Autodesk Inventor part; units mm, degrees
ref_plane "YZ Plane" through (0, 0, 0) normal (1, 0, 0) x (0, 1, 0)
ref_plane "XZ Plane" through (0, 0, 0) normal (0, 1, 0) x (-1, 0, 0)
ref_plane "XY Plane" through (0, 0, 0) normal (0, 0, 1) x (1, 0, 0)
sketch "Sketch1" plane through (0, 0, 0) normal (0, 1, 0) x (-1, 0, 0)
  line L0 (0, -5.4) -> (1.5, -5.4)
  line L1 (1.5, -5.4) -> (1.5, -8.1)
  line L2 (1.5, -8.1) -> (3.2, -8.1)
  line L3 (0, 0) -> (1.5, 0)
  line L4 (1.5, 0) -> (1.5, 2.7)
  line L5 (1.5, 2.7) -> (3.2, 2.7)
  line L6 (5, 0) -> (5, -5.4)
  line L7 (5, -5.4) -> (3.2, -8.1)
  line L8 (5, 0) -> (3.2, 2.7)
  line L9 (0, -20) -> (1.5, -20)
  line L10 (1.5, -20) -> (1.5, -17.3)
  line L11 (1.5, -17.3) -> (3.2, -17.3)
  line L12 (0, -25.4) -> (1.5, -25.4)
  line L13 (1.5, -25.4) -> (1.5, -28.1)
  line L14 (1.5, -28.1) -> (3.2, -28.1)
  line L15 (5, -20) -> (5, -25.4)
  line L16 (5, -25.4) -> (3.2, -28.1)
  line L17 (5, -20) -> (3.2, -17.3)
  line L18 (0, -5.4) -> (0, -20)
  line L19 (0, 0) -> (0, 7.3)
  line L20 (0, 7.3) -> (-5, 7.3)
  line L21 (0, -25.4) -> (0, -32.7)
  line L22 (0, -32.7) -> (-5, -32.7)
  line L23 (-5, -32.7) -> (-5, 7.3)
  dimension "d0" = 5.4
  dimension "d1" = 1.5
  dimension "d2" = 2.7
  dimension "d3" = 1.7
  dimension "d4" = 2.7
  dimension "d5" = 1.7
  dimension "d9" = 2.7
  dimension "d10" = 2.7
  dimension "d11" = 5.4
  dimension "d12" = 7.3
  dimension "d13" = 5
  dimension "d14" = 7.3
  dimension "d15" = 5
  dimension "d16" = 20
extrude "Extrusion1" add sketch "Sketch1" along normal blind 40
sketch "Sketch2" plane through (5, 0, 7.3) normal (1, 0, 0) x (0, 0, -1)
  line L0 (11.6599, 5) -> (8.3401, 5)
  line L1 (8.3401, 5) -> (6.6802, 7.875)
  line L2 (6.6802, 7.875) -> (8.3401, 10.75)
  line L3 (8.3401, 10.75) -> (11.6599, 10.75)
  line L4 (11.6599, 10.75) -> (13.3198, 7.875)
  line L5 (13.3198, 7.875) -> (11.6599, 5)
  line L6 (40, 0) -> (0, 0)
  line L7 (0, 0) -> (0, 40)
  line L8 (31.6599, 5) -> (28.3401, 5)
  line L9 (28.3401, 5) -> (26.6802, 7.875)
  line L10 (26.6802, 7.875) -> (28.3401, 10.75)
  line L11 (28.3401, 10.75) -> (31.6599, 10.75)
  line L12 (31.6599, 10.75) -> (33.3198, 7.875)
  line L13 (33.3198, 7.875) -> (31.6599, 5)
  line L14 (40, 0) -> (40, 40)
  line L15 (11.6599, 29.25) -> (8.3401, 29.25)
  line L16 (8.3401, 29.25) -> (6.6802, 32.125)
  line L17 (6.6802, 32.125) -> (8.3401, 35)
  line L18 (8.3401, 35) -> (11.6599, 35)
  line L19 (11.6599, 35) -> (13.3198, 32.125)
  line L20 (13.3198, 32.125) -> (11.6599, 29.25)
  line L21 (31.6599, 29.25) -> (28.3401, 29.25)
  line L22 (28.3401, 29.25) -> (26.6802, 32.125)
  line L23 (26.6802, 32.125) -> (28.3401, 35)
  line L24 (28.3401, 35) -> (31.6599, 35)
  line L25 (31.6599, 35) -> (33.3198, 32.125)
  line L26 (33.3198, 32.125) -> (31.6599, 29.25)
  line L27 (0, 40) -> (40, 40)
  point P0 (7.3, 0)
  point P1 (10, 7.875)
  point P2 (30, 7.875)
  point P3 (10, 32.125)
  point P4 (30, 32.125)
  dimension "d17" = 5.75
  dimension "d18" = 5
  dimension "d19" = 10
  dimension "d20" = 5.75
  dimension "d21" = 5
  dimension "d22" = 10
  dimension "d23" = 5.75
  dimension "d24" = 5.75
  dimension "d25" = 5
  dimension "d26" = 5
  dimension "d27" = 10
  dimension "d28" = 10
extrude "Extrusion2" cut sketch "Sketch2" against normal blind 2.5 contours L0 L1 L2 L3 L4 L5 | L8 L9 L10 L11 L12 L13 | L15 L16 L17 L18 L19 L20 | L21 L22 L23 L24 L25 L26
sketch "Sketch3" plane through (2.5, 0, 7.3) normal (1, 0, 0) x (0, 0, -1)
  circle A0 centre (30, 7.75) radius 1.375
  circle A1 centre (10, 7.75) radius 1.375
  circle A2 centre (10, 32.25) radius 1.375
  circle A3 centre (30, 32.25) radius 1.375
  point P0 (7.3, 0)
  dimension "d31" = 2.75
  dimension "d32" = 2.75
  dimension "d33" = 2.75
extrude "Extrusion3" cut sketch "Sketch3" against normal blind 20
sketch "Sketch4" plane through (0, 40, 0) normal (0, 1, 0) x (1, 0, 0)
  line L0 (5, -7.3) -> (5, 32.7)
  line L1 (5, -7.3) -> (-55, -7.3)
  line L2 (-55, -7.3) -> (-55, 32.7)
  line L3 (-55, 32.7) -> (5, 32.7)
  line L4 (5, 32.7) -> (5, -7.3)
  point P0 (0, 0)
  dimension "d36" = 60
extrude "Extrusion4" add sketch "Sketch4" along normal blind 5
sketch "Sketch5" plane through (0, 40, 0) normal (0, -1, 0) x (1, 0, 0)
  line L0 (-55, -32.7) -> (-55, 7.3)
  line L1 (-20.2, 0) -> (-55, 0)
  line L2 (-55, 0) -> (-55, -5.4)
  line L3 (-55, -5.4) -> (-20.2, -5.4)
  line L4 (-20.2, -5.4) -> (-20.2, 0)
  line L5 (0, -5.4) -> (0, -20)
  line L6 (-20.2, -20) -> (-55, -20)
  line L7 (-55, -20) -> (-55, -25.4)
  line L8 (-55, -25.4) -> (-20.2, -25.4)
  line L9 (-20.2, -25.4) -> (-20.2, -20)
  point P0 (0, 0)
  dimension "d39" = 5.4
  dimension "d40" = 20.2
  dimension "d41" = 5.4
extrude "Extrusion5" add sketch "Sketch5" along normal blind 1.5
sketch "Sketch6" plane through (-55, 40, 7.3) normal (-1, 0, 0) x (0, 0, 1)
  point P0 (-7.3, -40)
sketch "Sketch7" plane through (-55, 40, 7.3) normal (-1, 0, 0) x (0, 0, 1)
  point P0 (-7.3, -40)
sketch "Sketch8" plane through (0, 38.5, 0) normal (0, -1, 0) x (1, 0, 0)
  line L0 (-55, -32.7) -> (-55, 7.3)
  line L1 (-20.2, 2.7) -> (-55, 2.7)
  line L2 (-55, 2.7) -> (-55, -8.1)
  line L3 (-55, -8.1) -> (-20.2, -8.1)
  line L4 (-20.2, -8.1) -> (-20.2, 2.7)
  line L5 (-20.2, -17.3) -> (-55, -17.3)
  line L6 (-55, -17.3) -> (-55, -28.1)
  line L7 (-55, -28.1) -> (-20.2, -28.1)
  line L8 (-20.2, -28.1) -> (-20.2, -17.3)
  line L9 (-20.2, -20) -> (-55, -20)
  point P0 (0, 0)
  dimension "d44" = 10.8
  dimension "d45" = 10.8
  dimension "d46" = 2.7
extrude "Extrusion6" add sketch "Sketch8" along normal blind 1.7 contours L0 L1 L4 L3 | L0 L9 L8 L7
sketch "Sketch9" plane through (-55, 40, 7.3) normal (-1, 0, 0) x (0, 0, 1)
  line L0 (-7.3, -4.809) -> (-12.7, -4.809)
  line L1 (-12.7, -40) -> (-12.7, 0)
  line L2 (-4.6, -3.2) -> (-15.4, -3.2)
  line L3 (-12.7, -4.809) -> (-15.4, -3.2)
  line L4 (-15.4, -3.2) -> (-4.6, -3.2)
  line L5 (-4.6, -3.2) -> (-7.3, -4.809)
  point P0 (-7.3, -40)
  dimension "d49" = 5.4
extrude "Extrusion7" add sketch "Sketch9" against normal blind 34.8
sketch "Sketch10" plane through (-55, 40, -20) normal (0, 0, 1) x (1, 0, 0)
  line L0 (34.8, -3.2) -> (0, -3.2)
  line L1 (0, 0) -> (0, -3.2)
  line L2 (34.8, -3.2) -> (0, -3.2)
  line L3 (0, -3.2) -> (0, -1.5)
  line L4 (0, -1.5) -> (34.8, -1.5)
  line L5 (34.8, -1.5) -> (34.8, -3.2)
  point P0 (55, -40)
  dimension "d52" = 1.7
extrude "Extrusion8" add sketch "Sketch10" along normal blind 2.7
sketch "Sketch11" plane through (-55, 40, 7.3) normal (-1, 0, 0) x (0, 0, 1)
  line L0 (-24.6, -3.2) -> (-24.6, -1.5)
  line L1 (-35.4, -3.2) -> (-24.6, -3.2)
  line L2 (-24.6, -3.2) -> (-35.4, -3.2)
  line L3 (-27.3, -5) -> (-32.7, -5)
  line L4 (-32.7, -5) -> (-35.4, -3.2)
  line L5 (-24.6, -3.2) -> (-27.3, -5)
  line L6 (-27.3, 0) -> (-32.7, 0)
  point P0 (-7.3, -40)
  dimension "d55" = 5.4
  dimension "d56" = 5
extrude "Extrusion9" add sketch "Sketch11" against normal blind 34.8
sketch "Sketch12" plane through (0, 45, 0) normal (0, 1, 0) x (1, 0, 0)
  line L0 (-44.25, 4.3599) -> (-44.25, 1.0401)
  line L1 (-44.25, 1.0401) -> (-47.125, -0.6198)
  line L2 (-47.125, -0.6198) -> (-50, 1.0401)
  line L3 (-50, 1.0401) -> (-50, 4.3599)
  line L4 (-50, 4.3599) -> (-47.125, 6.0198)
  line L5 (-47.125, 6.0198) -> (-44.25, 4.3599)
  line L6 (-44.25, 24.3599) -> (-44.25, 21.0401)
  line L7 (-44.25, 21.0401) -> (-47.125, 19.3802)
  line L8 (-47.125, 19.3802) -> (-50, 21.0401)
  line L9 (-50, 21.0401) -> (-50, 24.3599)
  line L10 (-50, 24.3599) -> (-47.125, 26.0198)
  line L11 (-47.125, 26.0198) -> (-44.25, 24.3599)
  line L12 (-55, 25.4) -> (-20.2, 25.4)
  line L13 (-29.25, 4.3599) -> (-29.25, 1.0401)
  line L14 (-29.25, 1.0401) -> (-32.125, -0.6198)
  line L15 (-32.125, -0.6198) -> (-35, 1.0401)
  line L16 (-35, 1.0401) -> (-35, 4.3599)
  line L17 (-35, 4.3599) -> (-32.125, 6.0198)
  line L18 (-32.125, 6.0198) -> (-29.25, 4.3599)
  line L19 (-55, 32.7) -> (-55, -7.3)
  line L20 (5, 32.7) -> (-55, 32.7)
  line L21 (-55, -7.3) -> (5, -7.3)
  line L22 (-29.25, 24.3599) -> (-29.25, 21.0401)
  line L23 (-29.25, 21.0401) -> (-32.125, 19.3802)
  line L24 (-32.125, 19.3802) -> (-35, 21.0401)
  line L25 (-35, 21.0401) -> (-35, 24.3599)
  line L26 (-35, 24.3599) -> (-32.125, 26.0198)
  line L27 (-32.125, 26.0198) -> (-29.25, 24.3599)
  point P0 (0, 0)
  point P1 (-47.125, 2.7)
  point P2 (-47.125, 22.7)
  point P3 (-32.125, 2.7)
  point P4 (-32.125, 22.7)
  dimension "d59" = 5.75
  dimension "d60" = 5.75
  dimension "d61" = 5.75
  dimension "d62" = 5
  dimension "d63" = 5
  dimension "d64" = 20
  dimension "d67" = 10
  dimension "d69" = 10
  dimension "d70" = 10
extrude "Extrusion10" cut sketch "Sketch12" against normal blind 2.5
sketch "Sketch13" plane through (0, 42.5, 0) normal (0, 1, 0) x (1, 0, 0)
  circle A0 centre (-47.125, 2.7) radius 1.375
  circle A1 centre (-32.125, 2.7) radius 1.375
  circle A2 centre (-47.125, 22.7) radius 1.375
  circle A3 centre (-32.125, 22.7) radius 1.375
  line L0 (-44.25, 4.3599) -> (-44.25, 1.0401)
  line L1 (-29.25, 4.3599) -> (-29.25, 1.0401)
  line L2 (-29.25, 24.3599) -> (-29.25, 21.0401)
  line L3 (-35, 24.3599) -> (-32.125, 26.0198)
  line L4 (-35, 4.3599) -> (-32.125, 6.0198)
  line L5 (-50, 4.3599) -> (-47.125, 6.0198)
  line L6 (-44.25, 24.3599) -> (-44.25, 21.0401)
  line L7 (-50, 24.3599) -> (-47.125, 26.0198)
  point P0 (0, 0)
  dimension "d73" = 2.75
  dimension "d74" = 2.75
  dimension "d75" = 2.75
  dimension "d76" = 2.75
  dimension "d77" = 2.875
  dimension "d78" = 2.875
  dimension "d79" = 2.875
  dimension "d80" = 2.875
  dimension "d81" = 2.875
  dimension "d82" = 2.875
  dimension "d83" = 2.875
  dimension "d84" = 2.875
extrude "Extrusion11" cut sketch "Sketch13" against normal blind 20
properties part number "slotmountingPlate_dualcorner_m3"
Read the model definition and answer for the solid it produces. Units are mm, in the model's axes. A direction names the side the tool comes from. Coordinates: 2 decimals unless noted, no trailing zeros. Loops run counter-clockwise (first coordinate to the right, second up) from the corner with the lowest first, then second, coordinate; pieces in that order, holes last. Notation, with made-up numbers: (-8.75, 31.25) - (30.25, 31.25) arc R27 cw to (30.25, 69.25) - close; hole circle Ø11 at (40.5, 2.25). An arc over 180 degrees is marked (long way). Answer in a Markdown table with one row per item.
Q1. Find section C-C on z = -22.7. Count the separate pieces of the cut face and the enclosed holes in it, plus the area to 3 significant figures.
Here are the results:
| item | result |
|---|---|
| separate pieces | 5 |
| enclosed holes | 0 |
| area | 734 mm^2 |
Q2. Find section A-A on y = 16. Write down the section's boundary in (x, z), plus the area to 3 significant figures.
Here are the results:
| item | result |
|---|---|
| outline | (-5, -25.4) - (-3.2, -28.1) - (-1.5, -28.1) - (-1.5, -25.4) - (0, -25.4) - (0, -32.7) - (5, -32.7) - (5, 7.3) - (0, 7.3) - (0, 0) - (-1.5, 0) - (-1.5, 2.7) - (-3.2, 2.7) - (-5, 0) - (-5, -5.4) - (-3.2, -8.1) - (-1.5, -8.1) - (-1.5, -5.4) - (0, -5.4) - (0, -20) - (-1.5, -20) - (-1.5, -17.3) - (-3.2, -17.3) - (-5, -20) - close |
| area | 282 mm^2 |
Q3. For faces 1 (the flat face through (-1.5, 20, -7)), 2 (the flat face through (3.77, 6.42, -0.22)), 3 (the flat face through (-2, 20, 2.7)), 4 (the flat face through (-20.2, 38, -3)), determine the directions among +Z, -Z, +X, -X, +Y, -Y from which every point of the face is accessible in a straight line to the end or side of a thin tool.
Here are the results:
| item | result |
|---|---|
| face 1 | -Y |
| face 2 | +X |
| face 3 | +Z, -X, -Y |
| face 4 | +Z, -Z, -Y |
Q4. Straight lines are drawn through the part: line 1 along Y through (x, z) = (0, -22.7) (3 decimals); line 2 along X through (y, z) = (36.5, -22.5); line 3 along Z through (x, y) = (-1, 20). For each, find the intervals that lie inside material, in ascending order. Write a range as [from, to].
Here are the results:
| item | result |
|---|---|
| line 1 | y = [0, 6.375], [9.125, 30.875], [33.625, 45] |
| line 2 | x = [-55, -48.49], [-45.76, -33.49], [-30.76, -20.2], [-5, 5] |
| line 3 | z = [-25.4, -20], [-5.4, 0] |
Q5. The mould has two halves that part along X. Classify faces 5 (the flat face through (-37.844, 35.887, -26.731)), 6 (the flat face through (-1, 20, -5.4)): pulls with the +X half, pulls with the -X half, needs draft (parallel to the pull), parting line crosses it, or undercut.
Here are the results:
| item | result |
|---|---|
| face 5 | needs draft |
| face 6 | undercut |
Q6. Find section B-B on x = -36. Write down the section's boundary in (y, z).
Here are the results:
| item | result |
|---|---|
| outline | (35, -25.4) - (36.8, -28.1) - (38.5, -28.1) - (38.5, -25.4) - (40, -25.4) - (40, -32.7) - (45, -32.7) - (45, 7.3) - (40, 7.3) - (40, 0) - (38.5, 0) - (38.5, 2.7) - (36.8, 2.7) - (35.19, 0) - (35.19, -5.4) - (36.8, -8.1) - (38.5, -8.1) - (38.5, -5.4) - (40, -5.4) - (40, -20) - (38.5, -20) - (38.5, -17.3) - (36.8, -17.3) - (35, -20) - close |
Q7. Given P1, Ø1.9, axis at x = -2, y = 14, coming from the +Z side; P2, Ø5, axis at y = 34.5, z = -10, coming from the -X side; P3, Ø1.7, axis at x = -47, z = -23.5, coming from the +Y side, each flat-ended and moving along its own axis, determine where each tip first touches the part or whether it passes through.
Here are the results:
| item | result |
|---|---|
| P1 | stops at z = 2.7 |
| P2 | stops at x = -3.6 |
| P3 | stops at y = 42.5 |
